Geometry: final body of the model. Coordinates: model frame, mm. Round coordinates to 2 decimals unless told otherwise and drop trailing zeros. Order: outer loops, then holes, each group sorted by start corner. A loop starts at its lowest first (then second) coordinate and runs counter-clockwise, first axis right, second up. Notation, with made-up numbers: (11, 61) -> (54, 61) arc R34 cw to (54, 100) -> close; hole circle Ø11 at (10, -8.5). An arc over 180 degrees is marked (long way). Put each result on its own line as item: value.
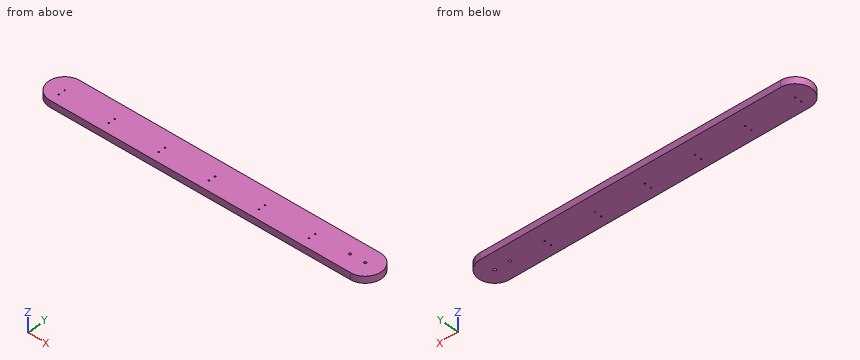
Autodesk Inventor part; units mm, degrees
ref_plane "Work Plane1" through (0, -2.5, 0) normal (0, 1, 0) x (-1, 0, 0)
ref_plane "YZ Plane" through (0, 0, 0) normal (1, 0, 0) x (0, 1, 0)
ref_plane "XY Plane" through (0, 0, 0) normal (0, 0, 1) x (1, 0, 0)
sketch "Sketch1" plane through (0, 0, 0) normal (0, 0, 1) x (1, 0, 0)
  line L0 (112.5, 0) -> (-112.5, 0) construction
  line L1 (112.5, 12) -> (-112.5, 12)
  line L2 (-112.5, -12) -> (112.5, -12)
  arc A0 (112.5, -12) -> (112.5, 12) centre (112.5, 0) ccw
  arc A1 (-112.5, 12) -> (-112.5, -12) centre (-112.5, 0) ccw
  point P0 (0, 0)
  dimension "d0" = 225
  dimension "d1" = 12
extrude "Extrusion1" add sketch "Sketch1" along normal blind 5
sketch "Sketch2" plane through (0, 0, 5) normal (0, 0, 1) x (1, 0, 0)
  arc A0 (112.5, -12) -> (112.5, 12) centre (112.5, 0) ccw
  point P0 (0, 0)
hole "Hole1" at (112.5, 0, 5) direction (0, 0, -1) diameter 1.9 end through all
sketch "Sketch3" plane through (0, 0, 5) normal (0, 0, 1) x (1, 0, 0)
  arc A0 (-112.5, 12) -> (-112.5, -12) centre (-112.5, 0) ccw
  circle A1 centre (112.5, 0) radius 0.95
  point P0 (0, 0)
  point P1 (75, 0)
  point P2 (37.5, 0)
  point P3 (0, 0)
  point P4 (-37.5, 0)
  point P5 (-75, 0)
  dimension "d33" = 37.5
  dimension "d34" = 37.5
  dimension "d35" = 37.5
  dimension "d36" = 37.5
hole "Hole2" at (-112.5, 0, 5) at (-75, 0, 5) at (-37.5, 0, 5) at (0, 0, 5) at (37.5, 0, 5) at (75, 0, 5) direction (0, 0, -1) diameter 1 end through all
sketch "Sketch4" plane through (0, 0, 5) normal (0, 0, 1) x (1, 0, 0)
  circle A0 centre (112.5, 0) radius 0.95
  point P0 (0, 0)
  point P1 (105, 0)
  point P2 (101.15, 0)
  dimension "d18" = 7.5
  dimension "d32" = 3.85
hole "Hole3" at (101.15, 0, 5) direction (0, 0, -1) diameter 1.8 end through all
ref_plane "Work Plane1" through (0, -2.5, 0) normal (0, 1, 0) x (-1, 0, 0)
mirror "Mirror1" about plane through (0, -2.5, 0) normal (0, 1, 0) of "Hole2"
sketch "Sketch5" plane through (0, 0, 5) normal (0, 0, 1) x (1, 0, 0)
  circle A0 centre (112.5, 0) radius 0.95
  point P0 (0, 0)
properties part number "Motor linkage"
1. Cut plane B-B on y = 6.75. Return loops of the section in (x, z).
Ans:
outline: (-122.42, 0) -> (122.42, 0) -> (122.42, 5) -> (-122.42, 5) -> close
2. Cut plane A-A on z = 3.7. State how many separate pieces and enclosed holes the cut face has, and give its area (3 significant figures).
Ans:
separate pieces: 1
enclosed holes: 14
area: 5,840 mm²
3. Contact query for a flat-ended pin moving along its axis: P1, Ø1.4, axis at x = 101.15, y = 0, coming from the -Z side. Output: stop coordinate, or through.
Ans:
P1: through
4. Material intervals for probe 1 along Y at (x, z) = (0, 2.7); probe 2 along X at (y, z) = (0.75, 2.55); probe 3 along X at (y, z) = (1, 2.7), sorted ascending.
Ans:
probe 1: -12 to -5.5, -4.5 to -0.5, 0.5 to 12
probe 2: -124.48 to 100.65, 101.65 to 111.92, 113.08 to 124.48
probe 3: -124.46 to 124.46
